Part model, mm, in its own coordinate system. A direction names the side the tool comes from. Round coordinates to 2 decimals unless told otherwise and drop trailing zeros. Loops run counter-clockwise (first coordinate to the right, second up) from the corner with the lowest first, then second, coordinate; pieces in that order, holes last. Notation, with made-up numbers: (65.5, 68.5) - (110.5, 68.5) arc R25 cw to (110.5, 96.5) - close; hole circle Ø5 at (39.5, -34). An arc over 180 degrees is marked (long way). Write each question's results on one line, items separated by ' | '. Start each with the question number.
(1) Flat gauge pins, fed straight in: P1, Ø1, axis at y = -9.5, z = -3.5, coming from the -X side; P2, Ø8, axis at x = 0, y = 0, coming from the -Z side; P3, Ø8, axis at x = 26, z = 15, coming from the +Y side. Where does each tip first touch, or does it go through?
(2) Mould opens along X. For faces 1 (the face through (-6, 8, -6)), 2 (the face through (26, -11, -12)), 3 (the face through (10.042, -2.307, -6.338)) say: released by +X, released by -X, zero draft, split by the parting line, or undercut.
(3) Tool access for faces 4 (the face through (18, -13.5, 0)), 5 (the face through (6, -8, 6)), 6 (the face through (20.505, -7.413, 15.225)), 7 (the face through (2.5, -2.7, -12.5)): list every direction of +Z, -Z, +X, -X, +Y, -Y with a clear straight run to the whole face (end or side of a thin tool).
(4) Cut at B-B, the plane z = 7. List the corners of the cut face in (x, y).
(5) Drill centre lines: L1, parallel to Z at x = 3, y = 8.25; L2, parallel to X at y = 0, z = 22; L3, parallel to X at y = -12.2, z = -15. Where is each one in solid material? Low to high.
(6) Cut at C-C, the plane y = 0. Give the number of separate pieces and of enclosed holes in the cut face, then the cut area to 3 significant figures.
(7) Cut at A-A, the plane z = -6.5. List the corners of the cut face in (x, y).
from build123d import *

# Parameters (mm, degrees)
SKETCH1_R           = 3.5
BOSS_EXTRUDE1_DEPTH = 25
SKETCH2_R           = 3
CUT_EXTRUDE1_DEPTH  = 51.460380498
SKETCH3_R           = 5.5
CUT_EXTRUDE2_DEPTH  = 49.334770094
SKETCH5_W           = 10
SKETCH5_H           = 12.5
FILLET3_R           = 1
FILLET4_R           = 1


with BuildPart() as part:
    # Sketch1 → Boss-Extrude1 (new, symmetric)
    with BuildSketch(Plane.XY):
        with BuildLine():
            Line((0, -13.5), (37, -13.5))
            Line((37, -13.5), (37, -8.5))
            Line((37, -8.5), (9.682458366, -2.5))
            ThreePointArc((9.682458366, -2.5), (-6.123724357, 7.90569415), (0, -10))
            Line((0, -10), (0, -13.5))
        make_face()
        Circle(SKETCH1_R, mode=Mode.SUBTRACT)
    extrude(amount=BOSS_EXTRUDE1_DEPTH, both=True)

    # Sketch2 → Cut-Extrude1 (cut, through all)
    with BuildSketch(Plane.XZ.offset(13.5)):
        with Locations(Location((26, 15, 0), (0, 0, 270))):
            Circle(SKETCH2_R)
        with Locations(Location((26, -15, 0), (0, 0, 270))):
            Circle(SKETCH2_R)
    extrude(amount=-CUT_EXTRUDE1_DEPTH, mode=Mode.SUBTRACT)

    # Sketch3 → Cut-Extrude2 (cut, through all)
    with BuildSketch(Plane(origin=(0, -8.5, 0), x_dir=(-1, 0, 0), z_dir=(0, -1, 0))):
        with Locations(Location((-26, 15, 0), (0, 0, 90))):
            Circle(SKETCH3_R)
        with Locations(Location((-26, -15, 0), (0, 0, 90))):
            Circle(SKETCH3_R)
    extrude(amount=-CUT_EXTRUDE2_DEPTH, mode=Mode.SUBTRACT)

    # Sketch5 → Cut-Revolve1 (revolve, cut)
    with BuildSketch(Plane(origin=(0, 0, 0), x_dir=(1, 0, 0), z_dir=(0, 1, 0)), mode=Mode.PRIVATE) as cut_revolve1_sk:
        with Locations((-5, 18.75)):
            Rectangle(SKETCH5_W, SKETCH5_H)
        with Locations((-5, -6.25)):
            Rectangle(SKETCH5_W, SKETCH5_H)
    revolve(cut_revolve1_sk.sketch.rotate(Axis((0, 0, -25), (0, 0, 1)), 180), axis=Axis((0, 0, -25), (0, 0, 1)), mode=Mode.SUBTRACT)

    # Fillet3
    fillet3_edges = [part.edges().sort_by_distance(p)[0] for p in [
        (9.682458366, -2.5, -6.25),
        (0, -10, -6.25),
        (9.682458366, -2.5, 18.75),
        (0, -10, 18.75),
    ]]
    fillet(fillet3_edges, radius=FILLET3_R)

    # Fillet4
    fillet4_edges = [part.edges().sort_by_distance(p)[0] for p in [
        (0, -12.227225575, 25),
        (-0.261451054, -10.280251288, 25),
        (-6.136482738, 7.895795058, 25),
        (10.03584865, -2.298357368, 25),
        (0, -10, -18.75),
        (0, -11.75, -25),
        (23.341229183, -5.5, -25),
        (6.123724357, -7.90569415, -25),
        (9.682458366, -2.5, -18.75),
        (37, -11, -25),
        (37, -11, 25),
        (37, -8.5, 0),
        (25.999999792, -6.083969958, -9.5),
        (25.999999792, -6.083969958, 20.5),
        (23.823868621, -5.606006487, 25),
        (0, -10, 6.25),
        (9.682458366, -2.5, 6.25),
    ]]
    fillet(fillet4_edges, radius=FILLET4_R)


solid = part.part
A:
1) P1: x = -4.36 | P2: z = -12.5 | P3: y = -8.5
2) face 1: split by the parting line | face 2: undercut | face 3: released by +X
3) face 4: +Z, -Z, +X, -X, -Y | face 5: -X, +Y | face 6: +Y | face 7: -Z, -X, +Y
4) outline: (0, -13.5) - (37, -13.5) - (37, -9.3) arc R1 ccw to (36.21, -8.33) - (10.58, -2.7) arc R1 ccw to (9.43, -3.34) arc R10 cw to (0.91, -9.96) arc R1 ccw to (0, -10.95) - close
5) L1: -12.5 to 0, 12.5 to 25 | L2: -10 to -3.5, 3.5 to 10 | L3: 0 to 23, 29 to 37
6) separate pieces: 4 | enclosed holes: 0 | area: 325 mm2
7) outline: (-0.91, -9.96) arc R1 cw to (0, -10.95) - (0, -13.5) - (37, -13.5) - (37, -9.3) arc R1 ccw to (36.21, -8.33) - (10.65, -2.71) arc R1 cw to (9.87, -1.58) arc R10 ccw (long way) to start; hole circle Ø7 at (0, 0)
